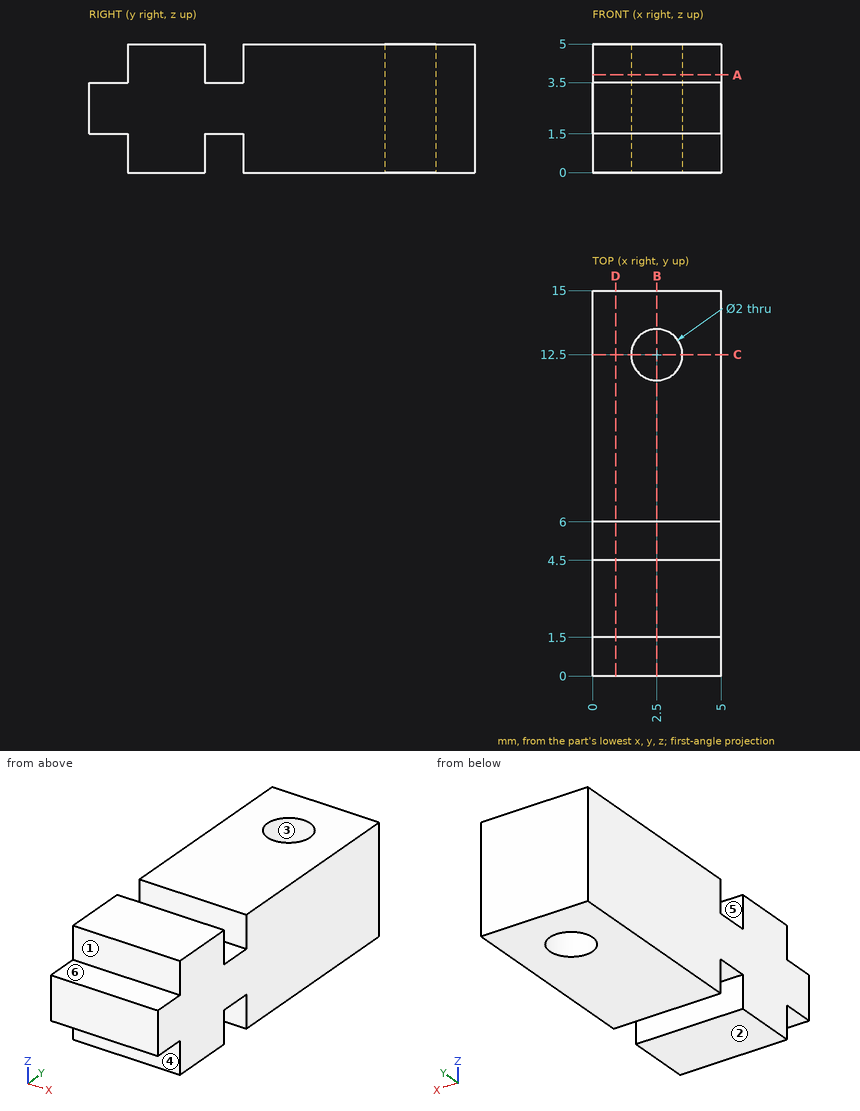
For this review, use the dimensioned drawing (mm, ordinates from the lowest corner) and the shaded views. A direction names the side the tool comes from. Coordinates: 2 decimals unless noted, no trailing zeros. Write each loop counter-clockwise with the first axis right and the second up, starting at its lowest first coordinate (ties: lowest second). Pieces come first, ordered by that corner, then holes. Notation, with made-up numbers: (56.25, 29) - (69.25, 29) arc R17 cw to (69.25, 60) - close; hole circle Ø6 at (-39.75, -36). An arc over 180 degrees is marked (long way). Answer as a JSON object with one key per item and string values. Group by question number.
1. Machinability: for the marked faces 4, 5 and 6, which of the approach directions +Z, -Z, +X, -X, +Y, -Y give a long, thin tool a straight path to every point of the face, cutting with its end or side? Answer none if there is none.
2. To check wall thickness, follow probe 1 along Y at (x, z) = (0.35, 4.6); probe 2 along Y at (x, z) = (2.5, 2.3); probe 3 along Z at (x, y) = (3.55, 5.5). State the ranges of each line that lie inside material, in increasing order.
3. Clearance check with flat-ended pins moving along their axes: pin 1 Ø1.6 at (x, y) = (2.5, 12.5) entering from -Z; pin 2 Ø1.2 at (x, z) = (3.5, 4.5) entering from -Y. State where each tip first meets the part, or that it passes through.
4. Add section A-A (z = 3.8). Give the boundary of the cut face in (x, y).
5. Add section B-B (x = 2.5). Give the boundary of the cut face in (y, z).
6. Add section D-D (x = 0.9). Give the boundary of the cut face in (y, z), plus the area to 3 significant figures.
7. Add section C-C (y = 12.5). Give the boundary of the cut face in (x, z), plus the area to 3 significant figures.
8. Mouldability with a two-part tool opening along Y and no side actions: class the marked faces 1, 2 and 3 as pulls with the +Y half, pulls with the -Y half, needs draft (parallel to the pull), parting line crosses it, or undercut.
Findings:
{
 "1": {"face 4": "-Z, +X, -X, -Y", "face 5": "+Z, +X, -X", "face 6": "+Z, +X, -X, -Y"},
 "2": {"probe 1": "1.5 to 4.5, 6 to 15", "probe 2": "0 to 11.5, 13.5 to 15", "probe 3": "1.5 to 3.5"},
 "3": {"pin 1": "through", "pin 2": "y = 1.5"},
 "4": {"outline": "(0, 1.5) - (5, 1.5) - (5, 4.5) - (0, 4.5) - close; (0, 6) - (5, 6) - (5, 15) - (0, 15) - close; hole circle Ø2 at (2.5, 12.5)"},
 "5": {"outline": "(0, 1.5) - (1.5, 1.5) - (1.5, 0) - (4.5, 0) - (4.5, 1.5) - (6, 1.5) - (6, 0) - (11.5, 0) - (11.5, 5) - (6, 5) - (6, 3.5) - (4.5, 3.5) - (4.5, 5) - (1.5, 5) - (1.5, 3.5) - (0, 3.5) - close; (13.5, 0) - (15, 0) - (15, 5) - (13.5, 5) - close"},
 "6": {"outline": "(0, 1.5) - (1.5, 1.5) - (1.5, 0) - (4.5, 0) - (4.5, 1.5) - (6, 1.5) - (6, 0) - (15, 0) - (15, 5) - (6, 5) - (6, 3.5) - (4.5, 3.5) - (4.5, 5) - (1.5, 5) - (1.5, 3.5) - (0, 3.5) - close", "area": "66.0 mm²"},
 "7": {"outline": "(0, 0) - (1.5, 0) - (1.5, 5) - (0, 5) - close; (3.5, 0) - (5, 0) - (5, 5) - (3.5, 5) - close", "area": "15.0 mm²"},
 "8": {"face 1": "pulls with the -Y half", "face 2": "needs draft", "face 3": "undercut"}
}
